Verification items for the finished model (mm, model axes). Coordinates: 2 decimals unless noted, no trailing zeros. Loops run counter-clockwise (first coordinate to the right, second up) from the corner with the lowest first, then second, coordinate; pieces in that order, holes last.
Q1. Material ranges on probe 1 along Z at (x, y) = (482.5, 3.4); probe 2 along X at (y, z) = (0.35, -106); probe 3 along Z at (x, y) = (398, 3.85), recorded low to high.
Q2. Go/stop test with flat-tipped pins: P1, Ø7, axis at x = 608.08, z = -78.09, coming from the +Y side; P2, Ø1.5, axis at y = 2.5, z = 144, coming from the +X side; P3, Ø2.5, axis at x = 386.5, y = 1.5, coming from the -Z side; P4, Ø1.5, axis at y = 3.5, z = -103, coming from the -X side. Record where each tip stops, or that it passes through.
Q3. Sectioned sample at A-A (z = 122). Enter the section's corners in (x, y), then the cut area to 3 significant figures.
Q4. Sectioned sample at C-C (z = -92). Enter the section's corners in (x, y), then the cut area to 3 significant figures.
Q5. Sectioned sample at B-B (y = 4.1). Count the separate pieces of the cut face and the enclosed holes in it, then the cut area to 3 significant figures.
Q6. Mould release check, pull along Z, two halves, no side actions. Record for faces 1 (the face through (611.455, 2.535, -75.936)), 2 (the face through (527, 5, 14)), 3 (the face through (366.79, 2.46, 148.67)): +Z half, -Z half, draft (parallel to the pull), parting line (faces both ways), or undercut.
```python
from build123d import *

# Parameters (mm, degrees)
RESSALTO_EXTRUS_O4_DEPTH = 5
ESBO_O2_R                = 2.5
CORTE_EXTRUS_O1_DEPTH    = 5
ESBO_O3_R                = 4
CORTE_EXTRUS_O2_DEPTH    = 5


with BuildPart() as part:
    # Esboço1 → Ressalto-extrusão4 (new body)
    with BuildSketch(Plane(origin=(0, 0, 0), x_dir=(1, 0, 0), z_dir=(0, 1, 0))):
        with BuildLine():
            Line((504.267355398, -155.796995794), (384.267355398, -155.796995794))
            ThreePointArc((384.267355398, -155.796995794), (366.589685869, -148.474665324), (359.267355398, -130.796995794))
            Line((359.267355398, -130.796995794), (359.267355398, 84.203004206))
            Line((359.267355398, 84.203004206), (399.267355398, 84.203004206))
            Line((399.267355398, 84.203004206), (399.267355398, 124.203004206))
            Line((399.267355398, 124.203004206), (649.267355398, 124.203004206))
            Line((649.267355398, 124.203004206), (649.267355398, 81.588187759))
            Line((649.267355398, 81.588187759), (689.267355398, 81.588187759))
            Line((689.267355398, 81.588187759), (689.267355398, -130.796995794))
            ThreePointArc((689.267355398, -130.796995794), (681.945024928, -148.474665324), (664.267355398, -155.796995794))
            Line((664.267355398, -155.796995794), (544.267355398, -155.796995794))
            Line((544.267355398, -155.796995794), (544.267355398, -115.796995794))
            Line((544.267355398, -115.796995794), (504.267355398, -115.796995794))
            Line((504.267355398, -115.796995794), (504.267355398, -155.796995794))
        make_face()
    extrude(amount=RESSALTO_EXTRUS_O4_DEPTH)

    # Esboço2 → Corte-extrusão1 (cut)
    with BuildSketch(Plane(origin=(0, 5, 0), x_dir=(1, 0, 0), z_dir=(0, 1, 0))):
        with Locations(Location((559.267355398, -100.796995794, 0), (0, 0, 270))):
            Circle(ESBO_O2_R)
        with Locations(Location((489.267355398, -100.796995794, 0), (0, 0, 270))):
            Circle(ESBO_O2_R)
        with Locations(Location((634.267355398, 66.588187759, 0), (0, 0, 270))):
            Circle(ESBO_O2_R)
        with Locations(Location((414.267355398, 69.203004206, 0), (0, 0, 270))):
            Circle(ESBO_O2_R)
    extrude(amount=-CORTE_EXTRUS_O1_DEPTH, mode=Mode.SUBTRACT)

    # Esboço3 → Corte-extrusão2 (cut)
    with BuildSketch(Plane(origin=(0, 5, 0), x_dir=(1, 0, 0), z_dir=(0, 1, 0))):
        with Locations(Location((608.081782449, -79.913221978, 0), (0, 0, 270))):
            Circle(ESBO_O3_R)
        with Locations(Location((484.081782449, -78.796995794, 0), (0, 0, 270))):
            Circle(ESBO_O3_R)
        with Locations(Location((484.081782449, 79.711850126, 0), (0, 0, 270))):
            Circle(ESBO_O3_R)
        with Locations(Location((608.081782449, 78.086778022, 0), (0, 0, 270))):
            Circle(ESBO_O3_R)
    extrude(amount=-CORTE_EXTRUS_O2_DEPTH, mode=Mode.SUBTRACT)


solid = part.part
```
Geometry check:
1. probe 1: z = -124.2 to -83.39, -76.04 to 75.12, 82.47 to 155.8
1. probe 2: x = 399.27 to 649.27
1. probe 3: z = -84.2 to 155.8
2. P1: passes through
2. P2: stops at x = 685.95
2. P3: stops at z = -84.2
2. P4: stops at x = 399.27
3. outline: (359.27, 0) - (504.27, 0) - (504.27, 5) - (359.27, 5) - close; (544.27, 0) - (689.27, 0) - (689.27, 5) - (544.27, 5) - close
3. area: 1,450 mm2
4. outline: (399.27, 0) - (649.27, 0) - (649.27, 5) - (399.27, 5) - close
4. area: 1,250 mm2
5. separate pieces: 1
5. enclosed holes: 8
5. area: 86,900 mm2
6. face 1: undercut
6. face 2: draft
6. face 3: +Z half
